Could you check a few things on this model? Use its own coordinates, in mm. A direction names the side the tool comes from. Coordinates: 2 decimals unless noted, no trailing zeros. Order: outer loops, then holes, each group sorted by start corner. A loop starts at its lowest first (then second) coordinate and runs counter-clockwise, first axis right, second up. Notation, with made-up numbers: (-16, 28) -> (9, 28) arc R24 ccw to (9, 66) -> close; hole circle Ø2 at (43, -21.5). An arc over 180 degrees is marked (long way). Put each result on its own line as item: value. Start each with the question number.
Q1. If we section it at A-A (y = 8.15): Count the separate pieces of the cut face and the enclosed holes in it, and give its area (3 significant figures).
Q2. Please list where these lines run through material, in increasing order: line 1 along X through (y, z) = (8.15, 3.3) (3 decimals); line 2 along Y through (x, z) = (2, 10) (3 decimals); line 3 along X through (y, z) = (7.5, 10) (3 decimals).
Q3. For faces 5 (the face through (21.75, 8.07, 3.28)), 6 (the face through (0, -1.125, 18)), 7 (the face through (37.78, 7.69, 27.47)), 8 (the face through (10.53, 14.42, 18.23)), 9 (the face through (19.237, 0.962, 3.278)), which set-ups out of +Z, -Z, +X, -X, +Y, -Y let a thin tool reach every point of the face, with its end or its side?
Q4. Will these pins go through, and if not, where does the flat tip stop? pin 1 (5 mm diameter, centred on x = -21.5, y = 3, fed in from -Z); pin 2 (3 mm diameter, centred on x = 13.5, z = 18.5, fed in from -Y) (3 decimals); pin 3 (13 mm diameter, centred on x = 2, y = 4.5, fed in from -Z); pin 4 (4 mm diameter, centred on y = 14.5, z = 20, fed in from -X).
Q5. We'd pull the mould along X, two halves only. Please class faces 1 (the face through (13.4, 4, 15)), 2 (the face through (-10.609, 14.336, 18.235)), 3 (the face through (18, 8, 1.75)), 4 (the face through (-18.25, 8.07, 3.28)): +X half, -X half, draft (parallel to the pull), parting line (faces both ways), or undercut.
Q6. If we section it at B-B (z = 8.5): Please give me the cut outline in (x, y) (3 decimals), and give its area (3 significant figures).
Q7. If we section it at C-C (x = -1.5): Please give me the cut outline in (y, z) (3 decimals).
Q8. If we section it at D-D (x = -20): Please give me the cut outline in (y, z).
from build123d import *

# Parameters (mm, degrees)
SKETCH_1_W                  = 30.26
SKETCH_1_H                  = 22
EXTRUDE_1_DEPTH             = 1.75
SKETCH_2_R                  = 1.75
EXTRUDE_2_DEPTH             = 3.1
EXTRUDE_3_DEPTH             = 27.15
SKETCH_4_R                  = 6.25
EXTRUDE_4_DEPTH             = 16
EXTRUDE_4_DIRECTION_2_REACH = 55.349
SKETCH_5_R                  = 3.5
EXTRUDE_5_DEPTH             = 17
CUT_EXTRUDE_1_DEPTH         = 17


with BuildPart() as part:
    # 草图1 → 凸台-拉伸1 (new body)
    with BuildSketch(Plane.XY):
        with Locations((0, 8.15)):
            Rectangle(SKETCH_1_W, SKETCH_1_H)
        Polygon((7.25, 16.3), (-7.25, 16.3), (-12.175, 11), (-12.175, 0), (12.175, 0), (12.175, 11), align=None, mode=Mode.SUBTRACT)
    extrude(amount=EXTRUDE_1_DEPTH)

    # 草图2 → 凸台-拉伸2 (add)
    with BuildSketch(Plane.XY.offset(1.75)):
        with BuildLine():
            Line((-15.13, 19.15), (15.13, 19.15))
            Line((15.13, 19.15), (23.231176295, 11.631666232))
            ThreePointArc((23.231176295, 11.631666232), (24.75, 8.15), (23.231176295, 4.668333768))
            Line((23.231176295, 4.668333768), (15.13, -2.85))
            Line((15.13, -2.85), (-15.13, -2.85))
            Line((-15.13, -2.85), (-23.231176295, 4.668333768))
            ThreePointArc((-23.231176295, 4.668333768), (-24.75, 8.15), (-23.231176295, 11.631666232))
            Line((-23.231176295, 11.631666232), (-15.13, 19.15))
        make_face()
        with Locations(Location((-20, 8.15, 0), (0, 0, 180))):
            Circle(SKETCH_2_R, mode=Mode.SUBTRACT)
        with Locations(Location((20, 8.15, 0), (0, 0, 180))):
            Circle(SKETCH_2_R, mode=Mode.SUBTRACT)
    extrude(amount=EXTRUDE_2_DEPTH)

    # 草图3 → 凸台-拉伸3 (add)
    with BuildSketch(Plane.XY.offset(4.85)):
        Polygon((13.4, -1.125), (-13.4, -1.125), (-13.4, 11.33280506), (-7.738856589, 17.425), (7.738856589, 17.425), (13.4, 11.33280506), align=None)
    extrude(amount=EXTRUDE_3_DEPTH)

    # 草图4 → 凸台-拉伸4 (add)
    with BuildSketch(Plane(origin=(13.4, 0, 0), x_dir=(0, 0, -1), z_dir=(1, 0, 0))):
        with Locations(Location((-24, 8.15, 0), (0, 0, 90))):
            Circle(SKETCH_4_R)
    extrude(amount=EXTRUDE_4_DEPTH)

    # 草图4 → 凸台-拉伸4 direction 2 (add, up to next)
    with BuildSketch(Plane(origin=(13.4, 0, 0), x_dir=(0, 0, -1), z_dir=(1, 0, 0)), mode=Mode.PRIVATE) as extrude_4_direction_2_sk1:
        with Locations(Location((-24, 8.15, 0), (0, 0, 90))):
            Circle(SKETCH_4_R)
    extrude_4_direction_2_tool1 = extrude(extrude_4_direction_2_sk1.sketch, amount=-EXTRUDE_4_DIRECTION_2_REACH, mode=Mode.PRIVATE) - part.part
    add(extrude_4_direction_2_tool1.solids().sort_by_distance((13.4, 8.15, 24))[0])

    # 草图5 → 凸台-拉伸5 (add)
    with BuildSketch(Plane(origin=(29.4, 0, 0), x_dir=(0, 0, -1), z_dir=(1, 0, 0))):
        with Locations(Location((-24, 8.15, 0), (0, 0, 90))):
            Circle(SKETCH_5_R)
    extrude(amount=EXTRUDE_5_DEPTH)

    # 草图6 → 切除-拉伸1 (cut)
    with BuildSketch(Plane(origin=(0, 0, 1.75), x_dir=(-1, 0, 0), z_dir=(0, 0, -1))):
        Polygon((-12.175, 11), (-12.175, 0), (12.175, 0), (12.175, 11), (7.25, 16.3), (-7.25, 16.3), align=None)
    extrude(amount=-CUT_EXTRUDE_1_DEPTH, mode=Mode.SUBTRACT)


solid = part.part
The answers:
1. separate pieces: 3
1. enclosed holes: 0
1. area: 775 mm^2
2. line 1: -24.75 to -21.75, -18.25 to -12.175, 12.175 to 18.25, 21.75 to 24.75
2. line 2: -1.125 to 0, 16.3 to 17.425
2. line 3: -13.4 to -12.175, 12.175 to 13.4
3. face 5: -Z
3. face 6: +Z, +X, -X, -Y
3. face 7: +X
3. face 8: +X, +Y
3. face 9: -Z, +X, -Y
4. pin 1: z = 1.75
4. pin 2: y = -1.125
4. pin 3: z = 0
4. pin 4: x = -12.32
5. face 1: +X half
5. face 2: -X half
5. face 3: draft
5. face 4: undercut
6. outline: (-13.4, -1.125) -> (13.4, -1.125) -> (13.4, 11.333) -> (7.739, 17.425) -> (-7.739, 17.425) -> (-13.4, 11.333) -> close; hole (-12.175, 0) -> (12.175, 0) -> (12.175, 11) -> (7.25, 16.3) -> (-7.25, 16.3) -> (-12.175, 11) -> close
6. area: 91.8 mm^2
7. outline: (-2.85, 0) -> (0, 0) -> (0, 18.75) -> (16.3, 18.75) -> (16.3, 0) -> (19.15, 0) -> (19.15, 4.85) -> (17.425, 4.85) -> (17.425, 32) -> (-1.125, 32) -> (-1.125, 4.85) -> (-2.85, 4.85) -> close
8. outline: (1.67, 1.75) -> (6.4, 1.75) -> (6.4, 4.85) -> (1.67, 4.85) -> close; (9.9, 1.75) -> (14.63, 1.75) -> (14.63, 4.85) -> (9.9, 4.85) -> close
